```python
from build123d import *

# Parameters (mm, degrees)
BOSS_EXTRUDE2_DEPTH     = 5
SKETCH2_W               = 18
SKETCH2_H               = 5
SKETCH2_W_2             = 33
CUT_EXTRUDE1_DEPTH      = 6
CUT_EXTRUDE1_DEPTH_BACK = 6


with BuildPart() as part:
    # Sketch1 → Boss-Extrude2 (new body, symmetric)
    with BuildSketch(Plane.XY):
        with BuildLine():
            Line((-23.57, 6), (-23.57, -12.112188076))
            ThreePointArc((-23.57, -12.112188076), (-13.807190445, -22.618830474), (0, -26.5))
            Line((0, -26.5), (0, 14))
            Line((0, 14), (-11, 14))
            Line((-11, 14), (-23.57, 6))
        make_face()
    boss_extrude2 = extrude(amount=BOSS_EXTRUDE2_DEPTH, both=True)

    # Mirror2: Boss-Extrude2 across plane
    add(boss_extrude2.mirror(Plane(origin=(0, 0, 0), x_dir=(0, 0, 1), z_dir=(1, 0, 0))))

    # Sketch1<6> → Cut-Revolve2 (revolve, cut)
    with BuildSketch(Plane.XY):
        with BuildLine():
            ThreePointArc((0, -26.5), (-13.807190445, -22.618830474), (-23.57, -12.112188076))
            Line((-23.57, -12.112188076), (-23.57, 6))
            Line((-23.57, 6), (-11, 14))
            Line((-11, 14), (0, 14))
            Line((0, 14), (0, 39.736431601))
            ThreePointArc((0, 39.736431601), (-39.736431601, 0), (0, -39.736431601))
            Line((0, -39.736431601), (0, -26.5))
        make_face()
    revolve(axis=Axis((0, 0, 0), (0, 1, 0)), mode=Mode.SUBTRACT)

    # Sketch2 → Cut-Extrude1 (cut, two sides)
    with BuildSketch(Plane.XY) as cut_extrude1_sk:
        with Locations((0, 8)):
            Rectangle(SKETCH2_W, SKETCH2_H)
        with Locations((0, 1.5)):
            Rectangle(SKETCH2_W_2, SKETCH2_H)
    extrude(amount=CUT_EXTRUDE1_DEPTH, mode=Mode.SUBTRACT)
    extrude(cut_extrude1_sk.sketch, amount=-CUT_EXTRUDE1_DEPTH_BACK, mode=Mode.SUBTRACT)


solid = part.part
```
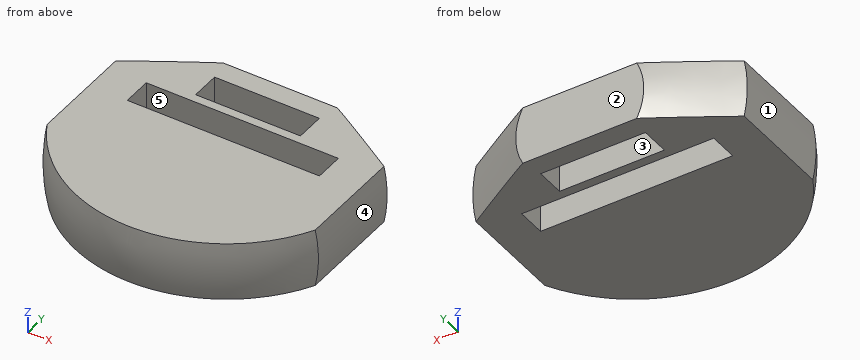
The listing builds one solid part. Answer for the finished solid, in the listing's coordinates (mm). Face numbers are marked on the shaded views. A direction names the side the tool comes from. Round coordinates to 2 decimals unless told otherwise and drop trailing zeros. Order: outer loops, then holes, each group sorted by start corner. A loop starts at its lowest first (then second) coordinate and runs counter-clockwise, first axis right, second up. Notation, with made-up numbers: (52.5, 61.25) - (64.5, 61.25) arc R26 cw to (64.5, 98.25) - close; hole circle Ø1 at (2, 37). An arc over 180 degrees is marked (long way). Put each result on its own line as item: value. Start each with the question number.
(1) Find section D-D (z = -1.25). State how many separate pieces and enclosed holes the cut face has, plus the area to 3 significant figures.
(2) Determine the mould class of the marked faces 1, 2 and 3 for opening direction X: released by +X, released by -X, zero draft, split by the parting line, or undercut.
(3) Find section B-B (x = -5). Give the vertices of the cut face in (y, z), plus the area to 3 significant figures.
(4) Given P1, Ø5, axis at y = -9.5, z = -4, coming from the +X side; P2, Ø5, axis at x = 2.5, z = 1, coming from the -Y side; P3, Ø1, axis at x = 10.5, z = 2, coming from the -Y side, each flat-ended and moving along its own axis, determine where each tip first touches the part or whether it passes through.
(5) For the marked faces 4 and 5, determine the directions among +Z, -Z, +X, -X, +Y, -Y from which every point of the face is accessible in a straight line to the end or side of a thin tool.
(6) Find section A-A (y = 8.5). Give the vertices of the cut face in (x, z).
(7) Straight lines are drawn through the part: probe 1 along X at (y, z) = (2, -0.25); probe 2 along Y at (x, z) = (-2, 2.75); probe 3 along Y at (x, z) = (5.5, -3). For each, find the intervals that lie inside material, in ascending order. Write a range as from..to.
(8) Find section C-C (y = 1.5). Give the vertices of the cut face in (x, z).
Reply:
1. separate pieces: 1
1. enclosed holes: 2
1. area: 1,360 mm^2
2. face 1: released by -X
2. face 2: zero draft
2. face 3: undercut
3. outline: (-25.54, -5) - (-1, -5) - (-1, 5) - (-25.54, 5) arc R26.02 ccw to start; (4, -5) - (5.5, -5) - (5.5, 5) - (4, 5) - close; (10.5, -5) - (14, -5) - (14, 5) - (10.5, 5) - close
3. area: 299 mm^2
4. P1: x = 23.52
4. P2: y = -26.5
4. P3: y = -24.46
5. face 4: +X, +Y, -Y
5. face 5: +Z, -Z
6. outline: (-18.99, -5) - (-9, -5) - (-9, 5) - (-18.99, 5) arc R19.64 ccw to start; (9, -5) - (18.99, -5) arc R19.64 ccw to (18.99, 5) - (9, 5) - close
7. probe 1: -23.57..-16.5, 16.5..23.57
7. probe 2: -26.28..-1, 4..5.5, 10.5..14
7. probe 3: -25.75..-1, 4..5.5, 10.5..14
8. outline: (-23.03, -5) - (-16.5, -5) - (-16.5, 5) - (-23.03, 5) arc R23.57 ccw to start; (16.5, -5) - (23.03, -5) arc R23.57 ccw to (23.03, 5) - (16.5, 5) - close
